Could you check a few things on this model? Use its own coordinates, in mm. A direction names the side the tool comes from. Give positions to 0.01 mm unless a question says otherwise; leave off trailing zeros. Loops run counter-clockwise (first coordinate to the right, second up) from the corner with the lowest first, then second, coordinate; pieces in that order, holes last. Notation, with made-up numbers: (84.5, -8.5) -> (122.5, -8.5) arc R13 ccw to (122.5, 1.5) -> close; hole circle Ø10 at (40.5, -28). An arc over 180 degrees is marked (long way). Write item = value, one per line. Start each with the question number.
1) On a 3-axis mill with a long thin cutter (end or side, diameter ignored), from which of +Z, -Z, +X, -X, +Y, -Y can I reach the whole of each face in a straight line? I mean faces 1 (the face through (47, 39, 0)), 2 (the face through (46.445, 39, -17)). Say none if no direction works.
2) I need wall thicknesses on probe 1 along Y at (x, z) = (36, -6); probe 2 along X at (y, z) = (68, -28.5); probe 3 along X at (y, z) = (74.75, -16.95). Which ranges of each line are inside material? Lowest first, please. Write a range as from..to.
3) I want a section at A-A (x = 40). List the corners of the cut face in (y, z) for me.
4) If we mould it in two halves opening along X, with no side actions, what happens to faces 3 (the face through (14.38, 3.451, -23.243)), 4 (the face through (14.38, 74.995, -23.243)), 5 (the face through (50.78, 76.49, -16.71)), 6 (the face through (28, 0, -17))? For each: +X half, -X half, draft (parallel to the pull), parting line (faces both ways), or undercut.
5) I want a section at C-C (x = 17.5). List the corners of the cut face in (y, z) for me, and give its area (3 significant figures).
6) I'm going to push a flat-ended pin straight in: pin 1 Ø8 at (y, z) = (19.5, -9) entering from -X. Where does the tip first touch, or does it pass through?
7) I want a section at D-D (y = 74). List the corners of the cut face in (x, z) for me.
8) I want a section at B-B (z = -16.95). List the corners of the cut face in (x, y) for me.
from build123d import *

# Parameters (mm, degrees)
SKETCH2_R           = 7.93
BOSS_EXTRUDE1_DEPTH = 78.59
FILLET1_R           = 7
CUT_EXTRUDE1_DEPTH  = 86.59
FILLET2_R           = 7


with BuildPart() as part:
    # Sketch2 → Boss-Extrude1 (new body)
    with BuildSketch(Plane(origin=(0, 0, 0), x_dir=(1, 0, 0), z_dir=(0, 1, 0))):
        with BuildLine():
            Line((-0.121305042, 14), (-0.121305042, 19.9))
            ThreePointArc((-0.121305042, 19.9), (3.979200021, 29.799494937), (13.878694958, 33.9))
            Line((13.878694958, 33.9), (52.778694958, 33.9))
            Line((52.778694958, 33.9), (52.778694958, 0))
            Line((52.778694958, 0), (13.878694958, 0))
            ThreePointArc((13.878694958, 0), (3.979200021, 4.100505063), (-0.121305042, 14))
        make_face()
        with Locations(Location((19.205687065, 16.95, 0), (0, 0, 270))):
            Circle(SKETCH2_R, mode=Mode.SUBTRACT)
    extrude(amount=BOSS_EXTRUDE1_DEPTH)

    # Fillet1
    fillet1_edges = [part.edges().sort_by_distance(p)[0] for p in [
        (52.778694958, 78.59, -16.95),
    ]]
    fillet(fillet1_edges, radius=FILLET1_R)

    # Sketch8 → Cut-Extrude1 (cut)
    with BuildSketch(Plane.XY):
        Polygon((46.445498075, 69.59), (46.445498075, 7), (13.878694958, 7), (-13.306366157, 7), (-13.306366157, 69.59), (-13.306366157, 71.500154521), (13.878694958, 71.500154521), (46.445498075, 71.500154521), align=None)
    extrude(amount=-CUT_EXTRUDE1_DEPTH, mode=Mode.SUBTRACT)

    # Fillet2
    fillet2_edges = [part.edges().sort_by_distance(p)[0] for p in [
        (52.778694958, 0, -16.95),
    ]]
    fillet(fillet2_edges, radius=FILLET2_R)


solid = part.part
Answer list:
q1.face_1 = +Z, +X, -X, +Y, -Y
q1.face_2 = +Z, -Z, -X
q2.probe_1 = 0..7, 71.5..78.59
q2.probe_2 = 46.45..52.78
q2.probe_3 = -0.12..11.28, 27.14..52.02
q3.outline = (0, -33.9) -> (7, -33.9) -> (7, 0) -> (0, 0) -> close; (71.5, -33.9) -> (78.59, -33.9) -> (78.59, 0) -> (71.5, 0) -> close
q4.face_3 = undercut
q4.face_4 = undercut
q4.face_5 = +X half
q4.face_6 = draft
q5.outline = (0, -33.9) -> (7, -33.9) -> (7, -24.69) -> (0, -24.69) -> close; (0, -9.21) -> (7, -9.21) -> (7, 0) -> (0, 0) -> close; (71.5, -33.9) -> (78.59, -33.9) -> (78.59, -24.69) -> (71.5, -24.69) -> close; (71.5, -9.21) -> (78.59, -9.21) -> (78.59, 0) -> (71.5, 0) -> close
q5.area = 259 mm^2
q6.pin_1 = 46.45
q7.outline = (-0.12, -19.9) arc R14 ccw to (13.88, -33.9) -> (52.35, -33.9) -> (52.35, 0) -> (13.88, 0) arc R14 ccw to (-0.12, -14) -> close; hole circle Ø15.86 at (19.21, -16.95)
q8.outline = (-0.12, 0) -> (11.28, 0) -> (11.28, 7) -> (-0.12, 7) -> close; (-0.12, 71.5) -> (11.28, 71.5) -> (11.28, 78.59) -> (-0.12, 78.59) -> close; (27.14, 0) -> (45.78, 0) arc R7 ccw to (52.78, 7) -> (52.78, 71.59) arc R7 ccw to (45.78, 78.59) -> (27.14, 78.59) -> (27.14, 71.5) -> (46.45, 71.5) -> (46.45, 7) -> (27.14, 7) -> close
